For this review, take the finished solid that the model builds, in its own axes (mm). Give positions to 0.01 mm unless a question says otherwise; leave off trailing zeros. Loops run counter-clockwise (first coordinate to the right, second up) from the corner with the lowest first, then second, coordinate; pieces in that order, holes last. Notation, with made-up numbers: (52.5, 38.5) -> (59.5, 38.5) arc R36 ccw to (59.5, 73.5) -> close; hole circle Ø8 at (44, -1). An arc over 180 degrees is marked (long way). One line per question, with ' | ' between items. Start each with the question number.
(1) Consider section A-A (z = -6.35). Write out the cut boundary in (x, y).
(2) Consider section C-C (z = -25.4). Write out the cut boundary in (x, y), and give its area (3 significant figures).
(3) Consider section B-B (y = 76.2). Write out the cut boundary in (x, z).
(4) Draft analysis for pull direction Y (two halves, no side actions). For faces 1 (the flat face through (2.54, 44, -75)), 2 (the cylindrical face through (1.252, 77.166, -144.79)), 3 (the cylindrical face through (1.252, 11.627, -5.18)), state which applies: +Y half, -Y half, draft (parallel to the pull), parting line (faces both ways), or undercut.
(5) Wall thickness on probe 1 along Z at (x, y) = (1.55, 12.7); probe 2 along Z at (x, y) = (1.7, 38.1); probe 3 along Y at (x, z) = (0.9, -50.8): over which ranges is each line inside the solid? List them lowest first.
Autodesk Inventor part; units mm, degrees
ref_plane "YZ Plane" through (0, 0, 0) normal (1, 0, 0) x (0, 1, 0)
ref_plane "XZ Plane" through (0, 0, 0) normal (0, 1, 0) x (-1, 0, 0)
ref_plane "XY Plane" through (0, 0, 0) normal (0, 0, 1) x (1, 0, 0)
sketch "Sketch1" plane through (0, 0, 0) normal (1, 0, 0) x (0, 1, 0)
  line L0 (0, 0) -> (88.9, 0)
  line L1 (88.9, 0) -> (88.9, -152.4)
  line L2 (88.9, -152.4) -> (0, -152.4)
  line L3 (0, -152.4) -> (0, 0)
  dimension "d0" = 88.9
  dimension "d1" = 152.4
extrude "Extrusion1" add sketch "Sketch1" along normal blind 2.54
sketch "Sketch2" plane through (2.54, 0, 0) normal (1, 0, 0) x (0, 0, -1)
  line L0 (0, 88.9) -> (0, 0)
  line L1 (0, 0) -> (152.4, 0)
  line L2 (152.4, 0) -> (152.4, 88.9)
  line L3 (152.4, 88.9) -> (0, 88.9)
  line L4 (6.35, 82.55) -> (6.35, 6.35) construction
  line L5 (6.35, 6.35) -> (146.05, 6.35) construction
  line L6 (146.05, 6.35) -> (146.05, 82.55) construction
  line L7 (146.05, 82.55) -> (6.35, 82.55) construction
  point P0 (6.35, 76.2)
  point P1 (6.35, 12.7)
  point P2 (146.05, 12.7)
  point P3 (146.05, 76.2)
  dimension "d4" = 6.35
  dimension "d5" = 12.7
  dimension "d6" = 12.7
  dimension "d7" = 12.7
  dimension "d8" = 12.7
hole "Hole1" at (2.54, 76.2, -6.35) at (2.54, 12.7, -6.35) at (2.54, 12.7, -146.05) at (2.54, 76.2, -146.05) direction (-1, 0, 0) diameter 3.175 depth 25.4 tip angle 118
sketch "Sketch3" plane through (2.54, 0, 0) normal (1, 0, 0) x (0, 0, -1)
  circle A0 centre (146.05, 12.7) radius 1.5875
  circle A1 centre (6.35, 76.2) radius 1.5875
  circle A2 centre (6.35, 12.7) radius 1.5875
  circle A3 centre (146.05, 76.2) radius 1.5875
  line L0 (0, 88.9) -> (0, 0) construction
  line L1 (0, 0) -> (152.4, 0) construction
  line L2 (152.4, 0) -> (152.4, 88.9) construction
  line L3 (152.4, 88.9) -> (0, 88.9) construction
  line L4 (-29.9282, 38.1) -> (171.8832, 38.1) construction
  point P0 (38.1, 38.1)
  point P1 (127, 38.1)
  point P2 (114.3, 38.1)
  point P3 (25.4, 38.1)
  dimension "d16" = 38.1
  dimension "d17" = 25.4
  dimension "d18" = 12.7
  dimension "d19" = 12.7
  dimension "d20" = 25.4
hole "Hole2" at (2.54, 38.1, -38.1) at (2.54, 38.1, -127) at (2.54, 38.1, -114.3) at (2.54, 38.1, -25.4) direction (-1, 0, 0) diameter 3.175 depth 25.4 tip angle 118
sketch "Sketch4" plane through (2.54, 0, 0) normal (1, 0, 0) x (0, 0, -1)
  line L0 (76.2, 87.9176) -> (76.2, -34.5253) construction
  circle A0 centre (38.1, 38.1) radius 1.5875 construction
  circle A1 centre (114.3, 38.1) radius 1.5875 construction
  line L1 (-38.8298, 38.1) -> (178.5898, 38.1) construction
  line L2 (-38.8298, 31.75) -> (180.6434, 31.75) construction
  line L3 (50.8, 85.0864) -> (50.8, -24.0085) construction
  line L4 (211.4025, 27.94) -> (-276.8587, 27.94) construction
  line L5 (-64.569, 19.05) -> (271.1941, 19.05) construction
  line L6 (-69.2198, 6.35) -> (225.3941, 6.35) construction
  circle A2 centre (50.8, 19.05) radius 1.5875
  circle A3 centre (50.8, 6.35) radius 1.5875
  point P0 (0, 0)
  point P1 (50.8, 31.75)
  dimension "d28" = 76.2
  dimension "d29" = 38.1
  dimension "d30" = 6.35
  dimension "d31" = 25.4
  dimension "d32" = 3.81
  dimension "d33" = 12.7
  dimension "d34" = 12.7
  dimension "d35" = 3.175
  dimension "d36" = 3.175
extrude "Extrusion2" cut sketch "Sketch4" against normal blind 25.4
properties part number "000201"
A:
1) outline: (0, 0) -> (2.54, 0) -> (2.54, 11.11) -> (0, 11.11) -> close; (0, 14.29) -> (2.54, 14.29) -> (2.54, 74.61) -> (0, 74.61) -> close; (0, 77.79) -> (2.54, 77.79) -> (2.54, 88.9) -> (0, 88.9) -> close
2) outline: (0, 0) -> (2.54, 0) -> (2.54, 36.51) -> (0, 36.51) -> close; (0, 39.69) -> (2.54, 39.69) -> (2.54, 88.9) -> (0, 88.9) -> close | area: 218 mm^2
3) outline: (0, -152.4) -> (2.54, -152.4) -> (2.54, -147.64) -> (0, -147.64) -> close; (0, -144.46) -> (2.54, -144.46) -> (2.54, -7.94) -> (0, -7.94) -> close; (0, -4.76) -> (2.54, -4.76) -> (2.54, 0) -> (0, 0) -> close
4) face 1: draft | face 2: undercut | face 3: undercut
5) probe 1: z = -152.4 to -147.64, -144.46 to -7.94, -4.76 to 0 | probe 2: z = -152.4 to -128.59, -125.41 to -115.89, -112.71 to -39.69, -36.51 to -26.99, -23.81 to 0 | probe 3: y = 0 to 4.76, 7.94 to 17.46, 20.64 to 88.9
